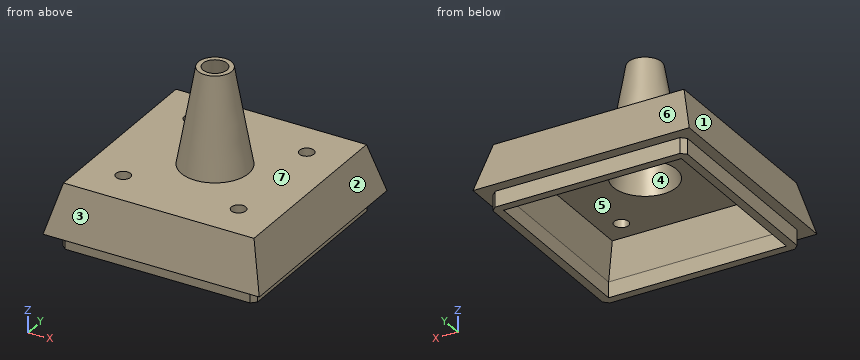
```python
from build123d import *

# Parameters (mm, degrees)
SKETCH004_W     = 40.5
SKETCH004_H     = 40.5
SKETCH004_W_2   = 37
SKETCH004_H_2   = 37
PAD001_DEPTH    = 3.25
SKETCH005_W     = 45
SKETCH005_H     = 45
PAD002_DEPTH    = 10
PAD002_TAPER    = 15
SKETCH006_W     = 37
SKETCH006_H     = 37
POCKET003_DEPTH = 7
POCKET003_TAPER = 15
SKETCH007_R     = 7
PAD003_DEPTH    = 20
PAD003_TAPER    = 10
SKETCH008_R     = 2.5
POCKET004_DEPTH = 25
POCKET004_TAPER = -10
SKETCH009_R     = 1.5
POCKET005_DEPTH = 13.251
CHAMFER001_SIZE = 1


with BuildPart() as part:
    # Sketch004 (on Face1 of Binder) → Pad001 (new body)
    with BuildSketch(Plane.XY.offset(37)):
        Rectangle(SKETCH004_W, SKETCH004_H)
        Rectangle(SKETCH004_W_2, SKETCH004_H_2, mode=Mode.SUBTRACT)
    extrude(amount=PAD001_DEPTH)

    # Sketch005 (on Face10 of Pad001) → Pad002 (join)
    with BuildSketch(Plane.XY.offset(40.25)):
        Rectangle(SKETCH005_W, SKETCH005_H)
    extrude(amount=PAD002_DEPTH, taper=PAD002_TAPER)

    # Sketch006 (on Face15 of Pad002) → Pocket003 (cut)
    with BuildSketch(Plane(origin=(0, 0, 40.25), x_dir=(1, 0, 0), z_dir=(0, 0, -1))):
        Rectangle(SKETCH006_W, SKETCH006_H)
    extrude(amount=-POCKET003_DEPTH, taper=POCKET003_TAPER, mode=Mode.SUBTRACT)

    # Sketch007 (on Face19 of Pocket003) → Pad003 (join)
    with BuildSketch(Plane.XY.offset(50.25)):
        Circle(SKETCH007_R)
    extrude(amount=PAD003_DEPTH, taper=PAD003_TAPER)

    # Sketch008 (on Face22 of Pad003) → Pocket004 (cut)
    with BuildSketch(Plane.XY.offset(70.25)):
        Circle(SKETCH008_R)
    extrude(amount=-POCKET004_DEPTH, taper=POCKET004_TAPER, mode=Mode.SUBTRACT)

    # Sketch009 (on Face19 of Pocket004) → Pocket005 (cut, through all)
    with BuildSketch(Plane.XY.offset(50.25)):
        with Locations((-12, 12)):
            Circle(SKETCH009_R)
        with Locations((12, 12)):
            Circle(SKETCH009_R)
        with Locations((-12, -12)):
            Circle(SKETCH009_R)
        with Locations((12, -12)):
            Circle(SKETCH009_R)
    extrude(amount=-POCKET005_DEPTH, mode=Mode.SUBTRACT)

    # Chamfer001
    chamfer001_edges = [part.edges().sort_by_distance(p)[0] for p in [
        (20.25, -20.25, 38.625),
        (-20.25, -20.25, 38.625),
        (-20.25, 20.25, 38.625),
        (20.25, 20.25, 38.625),
    ]]
    chamfer(chamfer001_edges, length=CHAMFER001_SIZE)


solid = part.part
```
Source: CAD feature listing. Evaluate the final solid. Frame: model axes, mm. Face numbers are marked on the shaded views. A direction names the side the tool comes from. Round coordinates to 2 decimals unless told otherwise and drop trailing zeros. Loops run counter-clockwise (first coordinate to the right, second up) from the corner with the lowest first, then second, coordinate; pieces in that order, holes last. Notation, with made-up numbers: (-36.75, 63) - (9.25, 63) arc R17 cw to (9.25, 86) - close; hole circle Ø8 at (23.25, -36). An arc over 180 degrees is marked (long way). Use CSV: the item, a comma, the result in double quotes.
Q1. Section query C-C, the plane z = 52.5. Output: boundary loops of the cut face in (x, y), then the cut area to 3 significant figures.
Reported:
outline,"circle Ø13.21 at (0, 0); hole circle Ø11.26 at (0, 0)"
area,"37.4 mm^2"
Q2. Mould query, pull axis X, two halves, no side actions, for the marked faces 1, 2, 3 and 4. Classes: pulls with the +X half, pulls with the -X half, needs draft (parallel to the pull), parting line crosses it, or undercut.
Reported:
face 1,"pulls with the -X half"
face 2,"pulls with the +X half"
face 3,"needs draft"
face 4,"undercut"
Q3. Reachability of the marked faces 5, 6 and 7 from +Z, -Z, +X, -X, +Y, -Y: full face, straight path, thin tool, end or side. Return the list, or none.
Reported:
face 5,"-Z"
face 6,"+Z, +X, -X, +Y"
face 7,"+Z"
Q4. Pin query (flat end, axial travel): pin 1 Ø2.5 at (x, z) = (-4.5, 38.5) entering from +Y; pin 2 Ø3.5 at (y, z) = (7.5, 39) entering from -X; pin 3 Ø12 at (y, z) = (-7, 65.5) entering from +X; pin 4 Ø4 at (x, y) = (-9, -12) entering from +Z. Return the tip coordinate at first contact, or that it passes through.
Reported:
pin 1,"y = 20.25"
pin 2,"x = -22.5"
pin 3,"x = 4.5"
pin 4,"z = 50.25"
Q5. Section query D-D, the plane z = 56. Output: boundary loops of the cut face in (x, y).
Reported:
outline,"circle Ø11.97 at (0, 0); hole circle Ø10.03 at (0, 0)"
Q6. Ray query, line 1 along Y through (x, z) = (-12, 48.6); line 2 along Y through (x, z) = (-12, 49.6); line 3 along Y through (x, z) = (-0.5, 39.5). Return the intervals inside material, ascending.
Reported:
line 1,"-20.26 to -13.5, -10.5 to 10.5, 13.5 to 20.26"
line 2,"-19.99 to -13.5, -10.5 to 10.5, 13.5 to 19.99"
line 3,"-20.25 to -18.5, 18.5 to 20.25"
Q7. Section query A-A, the plane y = 12. Give the number of separate pieces and of enclosed holes in the cut face, then the cut area to 3 significant figures.
Reported:
separate pieces,"3"
enclosed holes,"0"
area,"171 mm^2"
